Verification items for the finished model (mm, model axes). Round coordinates to 2 decimals unless told otherwise and drop trailing zeros. Order: outer loops, then holes, each group sorted by start corner. A loop starts at its lowest first (then second) coordinate and runs counter-clockwise, first axis right, second up.
Autodesk Inventor part; units mm, degrees
ref_plane "YZ Plane" through (0, 0, 0) normal (1, 0, 0) x (0, 1, 0)
ref_plane "XZ Plane" through (0, 0, 0) normal (0, 1, 0) x (-1, 0, 0)
ref_plane "XY Plane" through (0, 0, 0) normal (0, 0, 1) x (1, 0, 0)
sketch "Эскиз1" plane through (0, 0, 0) normal (0, 1, 0) x (-1, 0, 0)
  line L0 (-82.5, 225) -> (82.5, 225)
  line L1 (82.5, 225) -> (82.5, -225)
  line L2 (82.5, -225) -> (-82.5, -225)
  line L3 (-82.5, -225) -> (-82.5, 225)
  line L4 (-82.5, 225) -> (82.5, -225) construction
  line L5 (82.5, 225) -> (-82.5, -225) construction
  point P0 (0, 0)
  dimension "d0" = 165
  dimension "d1" = 450
extrude "Выдавливание1" add sketch "Эскиз1" along normal blind 4
sketch "Эскиз3" plane through (0, 0, 0) normal (0, -1, 0) x (1, 0, 0)
  circle A0 centre (42.3945, 182) radius 2
  circle A1 centre (-39.5136, 182) radius 2
  point P0 (0, 0)
extrude "Выдавливание3" cut sketch "Эскиз3" against normal blind 4
sketch "Эскиз4" plane through (0, 4, 0) normal (0, 1, 0) x (1, 0, 0)
  circle A0 centre (37.93, -81.5) radius 1.2889
  circle A1 centre (-37.0605, -72.5) radius 1.2889
  circle A2 centre (-37.0605, -141.5) radius 1.2889
  circle A3 centre (36.93, -141.5) radius 1.2889
  circle A4 centre (32.125, -13) radius 1.5
  circle A5 centre (69.125, -13) radius 1.5
  circle A6 centre (69.125, 24) radius 1.5
  circle A7 centre (32.125, 24) radius 1.5
  circle A8 centre (-32.125, 24) radius 1.5
  circle A9 centre (-69.125, 24) radius 1.5
  circle A10 centre (-69.125, -13) radius 1.5
  circle A11 centre (-32.125, -13) radius 1.5
  point P0 (0, 0)
extrude "Выдавливание4" cut sketch "Эскиз4" against normal blind 4
sketch "Эскиз5" plane through (0, 4, 0) normal (0, 1, 0) x (1, 0, 0)
  line L0 (-58.9065, 28.8404) -> (-29.5747, 28.8404)
  line L1 (-29.5747, 28.8404) -> (-29.5747, 43.2578)
  line L2 (-29.5747, 43.2578) -> (-58.9065, 43.2578)
  line L3 (-58.9065, 43.2578) -> (-58.9065, 28.8404)
  line L4 (-58.9065, 28.8404) -> (-29.5747, 43.2578) construction
  line L5 (-29.5747, 28.8404) -> (-58.9065, 43.2578) construction
  line L6 (-58.9065, -33.8129) -> (-29.5747, -33.8129)
  line L7 (-29.5747, -33.8129) -> (-29.5747, -19.3955)
  line L8 (-29.5747, -19.3955) -> (-58.9065, -19.3955)
  line L9 (-58.9065, -19.3955) -> (-58.9065, -33.8129)
  line L10 (-58.9065, -33.8129) -> (-29.5747, -19.3955) construction
  line L11 (-29.5747, -33.8129) -> (-58.9065, -19.3955) construction
  point P0 (0, 0)
  point P1 (-44.2406, 36.0491)
  point P2 (-44.2406, -26.6042)
extrude "Выдавливание5" cut sketch "Эскиз5" against normal blind 4
mirror "Зеркальное отражение1" about plane through (0, 0, 0) normal (1, 0, 0) of "Выдавливание5"
sketch "Эскиз6" plane through (0, 4, 0) normal (0, 1, 0) x (1, 0, 0)
  line L0 (71.4196, 151.6055) -> (-71.4196, 151.6055)
  line L1 (-71.4196, 151.6055) -> (-71.4196, 158.3091)
  line L2 (-71.4196, 158.3091) -> (71.4196, 158.3091)
  line L3 (71.4196, 158.3091) -> (71.4196, 151.6055)
  line L4 (71.4196, 151.6055) -> (-71.4196, 158.3091) construction
  line L5 (-71.4196, 151.6055) -> (71.4196, 158.3091) construction
  line L6 (71.4196, 203.7182) -> (-71.4196, 203.7182)
  line L7 (-71.4196, 203.7182) -> (-71.4196, 208.7265)
  line L8 (-71.4196, 208.7265) -> (71.4196, 208.7265)
  line L9 (71.4196, 208.7265) -> (71.4196, 203.7182)
  line L10 (71.4196, 203.7182) -> (-71.4196, 208.7265) construction
  line L11 (-71.4196, 203.7182) -> (71.4196, 208.7265) construction
  point P0 (0, 0)
  point P1 (0, 154.9573)
  point P2 (0, 206.2223)
extrude "Выдавливание6" cut sketch "Эскиз6" against normal blind 4
properties part number "bottom"
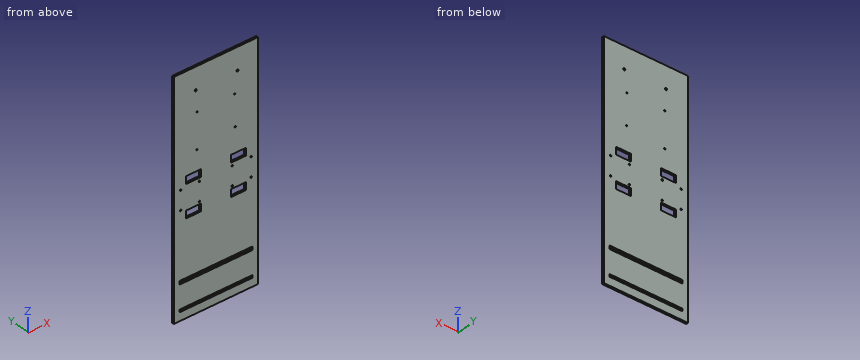
1) Scan lines: probe 1 along Z at (x, y) = (-62, 3.8); probe 2 along Z at (x, y) = (-57.5, 0.4); probe 3 along X at (y, z) = (3.1, 29). Record each from-to range of solid material in increasing order.
2) Sectioned sample at A-A on x = -25.5. Record the cut outline in (y, z).
3) Sectioned sample at B-B on y = 3.2. Count the separate pieces of the cut face and the enclosed holes in it, then the cut area to 3 significant figures.
Returned:
1. probe 1: z = -225 to -208.73, -203.72 to -158.31, -151.61 to 225
1. probe 2: z = -225 to -208.73, -203.72 to -158.31, -151.61 to -43.26, -28.84 to 19.4, 33.81 to 225
1. probe 3: x = -82.5 to -58.91, -29.57 to 29.57, 58.91 to 82.5
2. outline: (0, -225) - (4, -225) - (4, -208.73) - (0, -208.73) - close; (0, -203.72) - (4, -203.72) - (4, -158.31) - (0, -158.31) - close; (0, -151.61) - (4, -151.61) - (4, 225) - (0, 225) - close
3. separate pieces: 1
3. enclosed holes: 20
3. area: 70,800 mm2
